Design review of the part built by this model. Coordinates are the model's own, in mm. A direction names the side the tool comes from. Give positions to 0.01 mm unless a question says otherwise; leave off trailing zeros. Loops run counter-clockwise (first coordinate to the right, second up) from the corner with the lowest first, then second, coordinate; pieces in that order, holes last. Notation, with made-up numbers: (4.5, 82.25) -> (40.5, 82.25) arc R26 cw to (40.5, 112.25) -> close; hole circle Ø10 at (56.5, -5). An arc over 180 degrees is marked (long way). Use a Markdown table: item, result. Add a question column.
1. Add section B-B (x = -383.5). State the section outline as (y, z) points, and give its area (3 significant figures).
2. Draft analysis for pull direction Z (two halves, no side actions). For faces 1 (the flat face through (-9, -6, 100)), 2 (the flat face through (-350, -6, 110)), 3 (the cylindrical face through (-759.973, -5.6, 2.419)), state which applies: pulls with the +Z half, pulls with the -Z half, needs draft (parallel to the pull), parting line crosses it, or undercut.
3. For pin 1 Ø3 at (y, z) = (117.5, 60) entering from +X, flat-tipped, find the tip position at first contact; note if it passes through.
4. To check wall thickness, follow line 1 (Z direction, x = -505, y = 1.5); line 2 (Z direction, x = 13, y = 51.5); line 3 (X direction, y = 177, z = -38.5). State the ranges of each line that lie inside material, in increasing order.
5. Add section A-A (z = 0). State the section outline as (x, y) points.
6. Add section C-C (y = -56.5). State the section outline as (x, z) points, and give its area (3 significant figures).
7. For faces 4 (the cylindrical face through (749.976, -5.6, -2.199)), 5 (the flat face through (4, 400, 105)), 6 (the flat face through (341, -6, 110)), list the 3-axis set-ups (+Z, -Z, +X, -X, +Y, -Y) from which the entire face can be reached by the end or side of a thin tool; tool diameter is ignored.
8. Add section D-D (z = 142.5). State the section outline as (x, y) points, and give its area (3 significant figures).
```python
from build123d import *

# Parameters (mm, degrees)
PAD_DEPTH = 800


with BuildPart() as part:
    # Sketch → Pad (new body)
    with BuildSketch(Plane.XZ.offset(400)):
        with BuildLine():
            Line((-650.000001, 110), (-40.820946, 110))
            Line((-40.820946, 110), (0, 158.648546))
            Line((0, 158.648546), (40.820946, 110))
            Line((40.820946, 110), (649.999873, 110))
            ThreePointArc((649.999954, -110), (759.999874, 4.1e-05), (649.999873, 110))
            Line((-649.999998, -110), (649.999954, -110))
            ThreePointArc((-650.000001, 110), (-760.000001, -2e-06), (-649.999998, -110))
        make_face()
        with BuildLine():
            Line((-649.999999, 100), (649.999875, 100))
            ThreePointArc((650, -100), (749.999874, 6.3e-05), (649.999875, 100))
            Line((-650, -100), (650, -100))
            ThreePointArc((-649.999999, 100), (-750.000001, 1e-06), (-650, -100))
        make_face(mode=Mode.SUBTRACT)
    extrude(amount=-PAD_DEPTH)


solid = part.part
```
Taken from the geometry:
| question | item | result |
|---|---|---|
| 1 | outline | (-400, -110) -> (400, -110) -> (400, -100) -> (-400, -100) -> close; (-400, 100) -> (400, 100) -> (400, 110) -> (-400, 110) -> close |
| 1 | area | 16,000 mm^2 |
| 2 | face 1 | undercut |
| 2 | face 2 | pulls with the +Z half |
| 2 | face 3 | parting line crosses it |
| 3 | pin 1 | stops at x = 743.15 |
| 4 | line 1 | z = -110 to -100, 100 to 110 |
| 4 | line 2 | z = -110 to -100, 100 to 143.16 |
| 4 | line 3 | x = -753.04 to -742.29, 742.29 to 753.04 |
| 5 | outline | (-760, -400) -> (-750, -400) -> (-750, 400) -> (-760, 400) -> close; (750, -400) -> (760, -400) -> (760, 400) -> (750, 400) -> close |
| 6 | outline | (-650, -110) -> (650, -110) arc R110 ccw to (650, 110) -> (40.82, 110) -> (0, 158.65) -> (-40.82, 110) -> (-650, 110) arc R110 ccw to start; hole (-650, -100) -> (650, -100) arc R100 ccw to (650, 100) -> (-650, 100) arc R100 ccw to start |
| 6 | area | 34,600 mm^2 |
| 7 | face 4 | +Y, -Y |
| 7 | face 5 | +Z, -Z, +X, -X, +Y |
| 7 | face 6 | +Z, +X, +Y, -Y |
| 8 | outline | (-13.55, -400) -> (13.55, -400) -> (13.55, 400) -> (-13.55, 400) -> close |
| 8 | area | 21,700 mm^2 |
